Design review of the part built by this model. Coordinates are the model's own, in mm. A direction names the side the tool comes from. Give positions to 0.01 mm unless a question says otherwise; leave off trailing zeros. Order: outer loops, then holes, each group sorted by start corner. A loop starts at its lowest first (then second) coordinate and runs counter-clockwise, first axis right, second up. Notation, with made-up numbers: (61.5, 43) -> (107.5, 43) arc R23 ccw to (107.5, 67) -> close; hole circle Ø4 at (57.25, 17.25). An arc over 180 degrees is marked (long way). One line per item, written item: value.
from build123d import *

# Parameters (mm, degrees)
SKETCH1_W                          = 57.15
SKETCH1_H                          = 57.15
BOSS_EXTRUDE1_DEPTH                = 9.525
SKETCH2_W                          = 57.15
SKETCH2_H                          = 25.4
CUT_EXTRUDE1_DEPTH                 = 7.62
F_7_16_0_4375_DIAMETER_HOLE1_D     = 11.1125
F_7_16_0_4375_DIAMETER_HOLE1_DEPTH = 25.4
F_7_16_0_4375_DIAMETER_HOLE1_TIP   = 3.338531814
CUT_EXTRUDE3_DEPTH                 = 3.175
SKETCH9_W                          = 57.15
SKETCH9_H                          = 6.35
CUT_EXTRUDE4_DEPTH                 = 3.175


with BuildPart() as part:
    # Sketch1 → Boss-Extrude1 (new body)
    with BuildSketch(Plane(origin=(0, 0, 0), x_dir=(1, 0, 0), z_dir=(0, 1, 0))):
        Rectangle(SKETCH1_W, SKETCH1_H)
    extrude(amount=BOSS_EXTRUDE1_DEPTH)

    # Sketch2 → Cut-Extrude1 (cut)
    with BuildSketch(Plane(origin=(0, 9.525, 0), x_dir=(1, 0, 0), z_dir=(0, 1, 0))):
        with Locations((0, -9.525)):
            Rectangle(SKETCH2_W, SKETCH2_H)
    extrude(amount=-CUT_EXTRUDE1_DEPTH, mode=Mode.SUBTRACT)

    # 7/16 (0.4375) Diameter Hole1
    with Locations(Plane(origin=(0, 1.905, 0), x_dir=(1, 0, 0), z_dir=(0, 1, 0))):
        with Locations((0, -9.525)):
            Hole(F_7_16_0_4375_DIAMETER_HOLE1_D / 2, depth=F_7_16_0_4375_DIAMETER_HOLE1_DEPTH)
            with Locations((0, 0, -(F_7_16_0_4375_DIAMETER_HOLE1_DEPTH + F_7_16_0_4375_DIAMETER_HOLE1_TIP / 2))):  # 118° drill point
                Cone(0, F_7_16_0_4375_DIAMETER_HOLE1_D / 2, F_7_16_0_4375_DIAMETER_HOLE1_TIP, mode=Mode.SUBTRACT)

    # Sketch8 → Cut-Extrude3 (cut)
    with BuildSketch(Plane(origin=(0, 9.525, 0), x_dir=(1, 0, 0), z_dir=(0, 1, 0))):
        Polygon((0, 4.487899571), (28.575, 17.812640903), (28.575, 3.175), (0, 3.175), align=None)
    cut_extrude3 = extrude(amount=-CUT_EXTRUDE3_DEPTH, mode=Mode.SUBTRACT)

    # Mirror2: Cut-Extrude3 across plane
    add(cut_extrude3.mirror(Plane(origin=(0, 0, 0), x_dir=(0, 0, 1), z_dir=(1, 0, 0))), mode=Mode.SUBTRACT)

    # Sketch9 → Cut-Extrude4 (cut)
    with BuildSketch(Plane(origin=(0, 9.525, 0), x_dir=(1, 0, 0), z_dir=(0, 1, 0))):
        with Locations((0, -25.4)):
            Rectangle(SKETCH9_W, SKETCH9_H)
    extrude(amount=-CUT_EXTRUDE4_DEPTH, mode=Mode.SUBTRACT)


solid = part.part
Item 1: Add section C-C on x = -17. Give the boundary of the cut face in (y, z) (3 decimals), plus the area to 3 significant figures.
Returned:
outline: (0, -28.575) -> (9.525, -28.575) -> (9.525, -12.415) -> (6.35, -12.415) -> (6.35, -3.175) -> (1.905, -3.175) -> (1.905, 22.225) -> (6.35, 22.225) -> (6.35, 28.575) -> (0, 28.575) -> close
area: 301 mm²
Item 2: To check wall thickness, follow line 1 along Z through (x, y) = (0, 1.3) (3 decimals); line 2 along Z through (x, y) = (-3.5, 3.25) (3 decimals); line 3 along Y through (x, z) = (23, 24). State the ranges of each line that lie inside material, in increasing order. Write a range as from..to.
Returned:
line 1: -28.575..3.969, 15.081..28.575
line 2: -28.575..-3.175, 22.225..28.575
line 3: 0..6.35
Item 3: Add section B-B on z = 13.5. Give the boundary of the cut face in (x, y) (3 decimals), plus the area to 3 significant figures.
Returned:
outline: (-28.575, 0) -> (-3.882, 0) -> (-3.882, 1.905) -> (-28.575, 1.905) -> close; (3.882, 0) -> (28.575, 0) -> (28.575, 1.905) -> (3.882, 1.905) -> close
area: 94.1 mm²
Item 4: Add section D-D on y = 7.75. Give the boundary of the cut face in (x, z) (3 decimals), plus the area to 3 significant figures.
Returned:
outline: (-28.575, -28.575) -> (28.575, -28.575) -> (28.575, -17.813) -> (0, -4.488) -> (-28.575, -17.813) -> close
area: 996 mm²
Item 5: Draft analysis for pull direction Z (two halves, no side actions). For faces 4 (the flat face through (0, 4, 22.225)), 5 (the flat face through (0, 9.525, -19)), 6 (the flat face through (14.09, 7.96, -11.06)), state which applies: pulls with the +Z half, pulls with the -Z half, needs draft (parallel to the pull), parting line crosses it, or undercut.
Returned:
face 4: undercut
face 5: needs draft
face 6: pulls with the +Z half
Item 6: Add section A-A on y = 4.5. Give the boundary of the cut face in (x, z) (3 decimals).
Returned:
outline: (-28.575, -28.575) -> (28.575, -28.575) -> (28.575, -3.175) -> (-28.575, -3.175) -> close; (-28.575, 22.225) -> (28.575, 22.225) -> (28.575, 28.575) -> (-28.575, 28.575) -> close
Item 7: Clearance check with a flat-ended pin moving along its axis: P1, Ø1.9, axis at x = 4, z = 24, coming from the +Y side. State where the tip first meets the part, or that it passes through.
Returned:
P1: y = 6.35
Item 8: Machinability: for faces 1 (the flat face through (0, 6.35, -4)), 2 (the flat face through (0, 6.35, 25)), 3 (the flat face through (0, 4, -3.175)), which of the approach directions +Z, -Z, +X, -X, +Y, -Y give a long, thin tool a straight path to every point of the face, cutting with its end or side? Answer none if there is none.
Returned:
face 1: +Z, +Y
face 2: +Z, +X, -X, +Y
face 3: +X, -X, +Y
